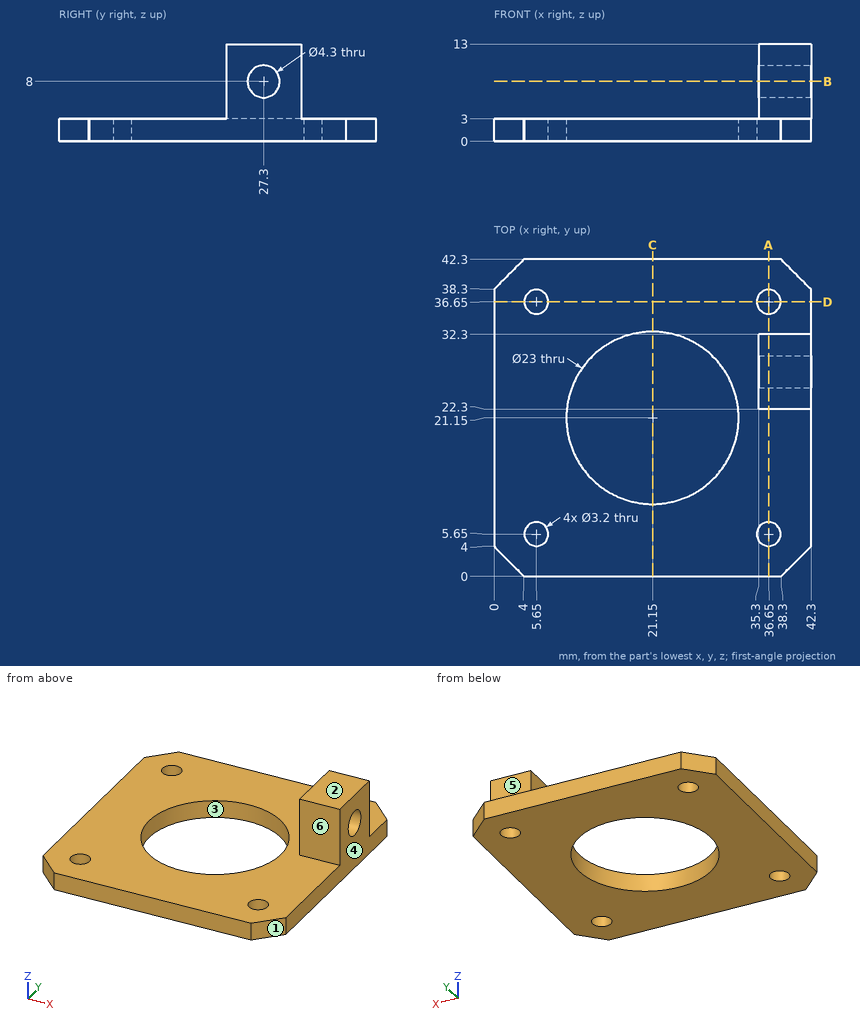
Geometry check sheet. Reference: drawing and pictorial views, mm from the part's lowest x, y, z. A direction names the side the tool comes from. Round coordinates to 2 decimals unless told otherwise and drop trailing zeros. Order: outer loops, then holes, each group sorted by start corner. A loop starts at its lowest first (then second) coordinate and runs counter-clockwise, first axis right, second up. Notation, with made-up numbers: (-12, 44.25) - (23, 44.25) arc R28 ccw to (23, 80.25) - close; hole circle Ø10 at (44, -9.5). An arc over 180 degrees is marked (long way). Use a Markdown table: item, result. Add a question column.
1) Section check C-C (x = 21.15). Record the cut outline in (y, z).
2) Gauge pin test, flat ends, axial feed: P1, Ø1, axis at x = 6, y = 13, coming from the +Z side; P2, Ø5, axis at y = 27.3, z = 8, coming from the -X side; P3, Ø2, axis at x = 37.5, z = 9.5, coming from the +Y side. Record the tip position at first contact, or that the pin passes through.
3) Section check A-A (x = 36.65). Record the cut outline in (y, z), then the cut area to 3 significant figures.
4) Section check D-D (y = 36.65). Record the cut outline in (x, z).
5) Section check B-B (z = 8). Record the cut outline in (x, y).
6) Set-up check for the marked faces 4, 5 and 6: record each of +Z, -Z, +X, -X, +Y, -Y from which the full face is reachable in a straight line by a thin tool's end or side.
7) Thickness scan on line 1 along Y through (x, z) = (5.65, 1.8); line 2 along Y through (x, z) = (38.5, 8); line 3 along Y through (x, z) = (21.15, 1.15). Record the ranges inside material, lowest first.
8) Mould release check, pull along Y, two halves, no side actions. Record for the marked faces 1, 2 and 3: released by +Y, released by -Y, zero draft, split by the parting line, or undercut.
Established:
| question | item | result |
|---|---|---|
| 1 | outline | (0, 0) - (9.65, 0) - (9.65, 3) - (0, 3) - close; (32.65, 0) - (42.3, 0) - (42.3, 3) - (32.65, 3) - close |
| 2 | P1 | z = 3 |
| 2 | P2 | x = 35.3 |
| 2 | P3 | y = 32.3 |
| 3 | outline | (0, 0) - (4.05, 0) - (4.05, 3) - (0, 3) - close; (7.25, 0) - (35.05, 0) - (35.05, 3) - (32.3, 3) - (32.3, 13) - (22.3, 13) - (22.3, 3) - (7.25, 3) - close; (38.25, 0) - (42.3, 0) - (42.3, 3) - (38.25, 3) - close; hole circle Ø4.3 at (27.3, 8) |
| 3 | area | 193 mm2 |
| 4 | outline | (0, 0) - (4.05, 0) - (4.05, 3) - (0, 3) - close; (7.25, 0) - (35.05, 0) - (35.05, 3) - (7.25, 3) - close; (38.25, 0) - (42.3, 0) - (42.3, 3) - (38.25, 3) - close |
| 5 | outline | (35.3, 22.3) - (42.3, 22.3) - (42.3, 25.15) - (35.3, 25.15) - close; (35.3, 29.45) - (42.3, 29.45) - (42.3, 32.3) - (35.3, 32.3) - close |
| 6 | face 4 | +Z, -Z, +X, +Y, -Y |
| 6 | face 5 | +Z, +X, -X, +Y |
| 6 | face 6 | +Z, +X, -X, -Y |
| 7 | line 1 | 0 to 4.05, 7.25 to 35.05, 38.25 to 42.3 |
| 7 | line 2 | 22.3 to 25.15, 29.45 to 32.3 |
| 7 | line 3 | 0 to 9.65, 32.65 to 42.3 |
| 8 | face 1 | released by -Y |
| 8 | face 2 | zero draft |
| 8 | face 3 | undercut |
